Part model, mm, in its own coordinate system. A direction names the side the tool comes from. Round coordinates to 2 decimals unless told otherwise and drop trailing zeros. Loops run counter-clockwise (first coordinate to the right, second up) from the corner with the lowest first, then second, coordinate; pieces in that order, holes last. Notation, with made-up numbers: (21, -28) -> (53, -28) arc R24 cw to (53, -8) -> close; hole circle Ø3 at (-23.5, -11). An arc over 180 degrees is marked (long way). Answer as a JSON object with one key per item and string values. Group by question number.
from build123d import *

# Parameters (mm, degrees)
SKETCH1_W           = 23
SKETCH1_H           = 12
BOSS_EXTRUDE1_DEPTH = 23
SKETCH2_W           = 12
SKETCH2_H           = 2.5
BOSS_EXTRUDE2_DEPTH = 5.5
CUT_EXTRUDE1_DEPTH  = 5
BOSS_EXTRUDE3_DEPTH = 4
SKETCH5_R           = 2.5
SKETCH5_R_2         = 1
BOSS_EXTRUDE4_DEPTH = 3
SKETCH7_R           = 0.6
BOSS_EXTRUDE8_DEPTH = 5


with BuildPart() as part:
    # Sketch1 → Boss-Extrude1 (new body)
    with BuildSketch(Plane(origin=(0, 0, 0), x_dir=(1, 0, 0), z_dir=(0, 1, 0))):
        Rectangle(SKETCH1_W, SKETCH1_H)
    extrude(amount=BOSS_EXTRUDE1_DEPTH)

    # Sketch2 → Boss-Extrude2 (add)
    with BuildSketch(Plane.ZY.offset(11.5)):
        with Locations((0, 17.25)):
            Rectangle(SKETCH2_W, SKETCH2_H)
    boss_extrude2 = extrude(amount=BOSS_EXTRUDE2_DEPTH)

    # Sketch3 → Cut-Extrude1 (cut)
    with BuildSketch(Plane(origin=(0, 18.5, 0), x_dir=(1, 0, 0), z_dir=(0, 1, 0))):
        with BuildLine():
            Line((-17, 0.6), (-15.3, 0.6))
            ThreePointArc((-15.3, 0.6), (-13.506719548, -0.11573221), (-15.416515139, -0.4))
            Line((-15.416515139, -0.4), (-17, -0.4))
            Line((-17, -0.4), (-17, 0.6))
        make_face()
    cut_extrude1 = extrude(amount=-CUT_EXTRUDE1_DEPTH, mode=Mode.SUBTRACT)

    # Mirror1: Boss-Extrude2, Cut-Extrude1 across plane
    add(boss_extrude2.mirror(Plane(origin=(0, 0, 0), x_dir=(0, 0, 1), z_dir=(1, 0, 0))))
    add(cut_extrude1.mirror(Plane(origin=(0, 0, 0), x_dir=(0, 0, 1), z_dir=(1, 0, 0))), mode=Mode.SUBTRACT)

    # Sketch4 → Boss-Extrude3 (add)
    with BuildSketch(Plane(origin=(0, 23, 0), x_dir=(1, 0, 0), z_dir=(0, 1, 0))):
        with BuildLine():
            ThreePointArc((0.25, -2.90473751), (11.5, 0), (0.25, 2.90473751))
            ThreePointArc((0.25, 2.90473751), (-3.5, 0), (0.25, -2.90473751))
        make_face()
    extrude(amount=BOSS_EXTRUDE3_DEPTH)

    # Sketch5 → Boss-Extrude4 (add)
    with BuildSketch(Plane(origin=(0, 27, 0), x_dir=(1, 0, 0), z_dir=(0, 1, 0))):
        with Locations((5.5, 0)):
            Circle(SKETCH5_R)
        with Locations((5.5, 0)):
            Circle(SKETCH5_R_2, mode=Mode.SUBTRACT)
    extrude(amount=BOSS_EXTRUDE4_DEPTH)

    # Sketch7 → Boss-Extrude8 (add)
    with BuildSketch(Plane(origin=(11.5, 0, 0), x_dir=(0, 0, -1), z_dir=(1, 0, 0))):
        with Locations((0, 5.5)):
            Circle(SKETCH7_R)
        with Locations((1.21, 5.5)):
            Circle(SKETCH7_R)
        with Locations((-1.21, 5.5)):
            Circle(SKETCH7_R)
    extrude(amount=BOSS_EXTRUDE8_DEPTH)


solid = part.part
Item 1: Drill centre lines: line 1 (Z direction, x = -14.5, y = 16.6); line 2 (X direction, y = 28.55, z = 0); line 3 (X direction, y = 15.25, z = 3.75). Where is each one in solid material? Low to high.
Item 2: Band-saw the part on C-C, the plane y = 10.75. List the corners of the cut face in (x, z).
Item 3: Drop flat-ended pins along their axis: pin 1 Ø1.2 at (x, z) = (14.5, 0) entering from -Y; pin 2 Ø6 at (y, z) = (8, 1.5) entering from +X; pin 3 Ø6 at (x, z) = (-4, -0.5) entering from +Y; pin 4 Ø1 at (x, y) = (13, 8) entering from -Z. Give the stop position or say it passes through.
Item 4: Band-saw the part on B-B, the plane x = 14.5. List the corners of the cut face in (y, z).
Item 5: Which spindle directions (+Z, -Z, +X, -X, +Y, -Y) get a long thin tool onto all of the face, cutting with end or side? Do faces 5 (the face through (16.5, 5.5, 0)), 6 (the face through (13, 16, 0)), 7 (the face through (11.5, 21, 0)), 8 (the face through (-11.5, 8, 0)). Say none if no direction does.
Item 6: Two-plate mould, pull along Z, no slides. Class faces 1 (the face through (0, 11, 6)), 2 (the face through (-11.5, 21, 0)), 3 (the face through (13.965, 4.914, -1.08)), 4 (the face through (-3.5, 25, -0.1)): pulls with the +Z half, pulls with the -Z half, needs draft (parallel to the pull), parting line crosses it, or undercut.
Item 7: Band-saw the part on A-A, the plane x = -14.5. List the corners of the cut face in (y, z).
Item 8: Band-saw the part on D-D, the plane z = -3.5. List the corners of the cut face in (x, y).
Entries:
{
 "1": {"line 1": "-6 to -1, 1 to 6", "line 2": "3 to 4.5, 6.5 to 8", "line 3": "-11.5 to 11.5"},
 "2": {"outline": "(-11.5, -6) -> (11.5, -6) -> (11.5, 6) -> (-11.5, 6) -> close"},
 "3": {"pin 1": "y = 4.9", "pin 2": "x = 16.5", "pin 3": "y = 27", "pin 4": "through"},
 "4": {"outline": "circle Ø1.2 at (5.5, -1.21); circle Ø1.2 at (5.5, 0); circle Ø1.2 at (5.5, 1.21); (16, -6) -> (18.5, -6) -> (18.5, -1) -> (16, -1) -> close; (16, 1) -> (18.5, 1) -> (18.5, 6) -> (16, 6) -> close"},
 "5": {"face 5": "+Z, -Z, +X, -Y", "face 6": "+Z, -Z, +X", "face 7": "+Z, -Z, +X, +Y", "face 8": "+Z, -Z, -X, -Y"},
 "6": {"face 1": "pulls with the +Z half", "face 2": "needs draft", "face 3": "undercut", "face 4": "parting line crosses it"},
 "7": {"outline": "(16, -6) -> (18.5, -6) -> (18.5, -1) -> (16, -1) -> close; (16, 1) -> (18.5, 1) -> (18.5, 6) -> (16, 6) -> close"},
 "8": {"outline": "(-17, 16) -> (-11.5, 16) -> (-11.5, 0) -> (11.5, 0) -> (11.5, 16) -> (17, 16) -> (17, 18.5) -> (11.5, 18.5) -> (11.5, 23) -> (10.37, 23) -> (10.37, 27) -> (0.63, 27) -> (0.63, 23) -> (-11.5, 23) -> (-11.5, 18.5) -> (-17, 18.5) -> close"}
}
